Read the model definition and answer for the solid it produces. Units are mm, in the model's axes. A direction names the side the tool comes from. Give positions to 0.01 mm unless a question says otherwise; leave off trailing zeros. Loops run counter-clockwise (first coordinate to the right, second up) from the corner with the lowest first, then second, coordinate; pieces in that order, holes last. Notation, with made-up numbers: (9, 13.25) -> (30, 13.25) arc R30 cw to (30, 49.25) -> close; hole circle Ø1 at (-16.75, 30). An arc over 180 degrees is marked (long way). Return JSON: item names as keys, results as strings. Group by question number.
from build123d import *

# Parameters (mm, degrees)
SKETCH1_R           = 400
BOSS_EXTRUDE1_DEPTH = 200
BOSS_EXTRUDE2_START = -10
SKETCH2_R           = 82.5
SKETCH2_R_2         = 75.5
BOSS_EXTRUDE2_DEPTH = 33
CUT_EXTRUDE1_START  = -432
SKETCH2_2_R         = 75.5
CUT_EXTRUDE1_DEPTH  = 432
SKETCH3_R           = 275.958825931
CUT_EXTRUDE3_DEPTH  = 175
FILLET2_R           = 10


with BuildPart() as part:
    # Sketch1 → Boss-Extrude1 (new body)
    with BuildSketch(Plane(origin=(0, 0, 0), x_dir=(1, 0, 0), z_dir=(0, 1, 0))):
        with Locations(Location((0, 0, 0), (0, 0, 270))):
            Circle(SKETCH1_R)
    extrude(amount=BOSS_EXTRUDE1_DEPTH)

    # Sketch2 → Boss-Extrude2 (add)
    with BuildSketch(Plane.XY.offset(400).offset(BOSS_EXTRUDE2_START)):
        with Locations(Location((0, 104.933431854, 0), (0, 0, 180))):
            Circle(SKETCH2_R)
        with Locations(Location((0, 104.933431854, 0), (0, 0, 180))):
            Circle(SKETCH2_R_2, mode=Mode.SUBTRACT)
    extrude(amount=BOSS_EXTRUDE2_DEPTH)

    # Sketch2_2 → Cut-Extrude1 (cut)
    with BuildSketch(Plane.XY.offset(400).offset(CUT_EXTRUDE1_START)):
        with Locations((0, 104.933431854)):
            Circle(SKETCH2_2_R)
    extrude(amount=CUT_EXTRUDE1_DEPTH, mode=Mode.SUBTRACT)

    # Sketch3 → Cut-Extrude3 (cut)
    with BuildSketch(Plane(origin=(0, 200, 0), x_dir=(1, 0, 0), z_dir=(0, 1, 0))):
        with Locations(Location((0, 0, 0), (0, 0, 270))):
            Circle(SKETCH3_R)
    extrude(amount=-CUT_EXTRUDE3_DEPTH, mode=Mode.SUBTRACT)

    # Fillet2
    fillet2_edges = [part.edges().sort_by_distance(p)[0] for p in [
        (82.5, 104.933431854, 391.399731732),
    ]]
    fillet(fillet2_edges, radius=FILLET2_R)


solid = part.part
1. Flat-ended cylindrical pins translate along their axes: pin 1 Ø1.5 at (y, z) = (149.5, -123) entering from +X; pin 2 Ø3 at (x, y) = (-198, 95.5) entering from -Z; pin 3 Ø6 at (y, z) = (159.5, 250) entering from +X. Find the tip coordinate at first contact, or state that the pin passes through.
2. Section B-B on x = 132 is taken. Determine the outline of the cut face in (y, z).
3. Which of the six approach directions +Z, -Z, +X, -X, +Y, -Y give full straight-line access (tool end or side, diameter ignored) to faces 5 (the flat face through (6, 0, -6)), 6 (the cylindrical face through (4.98, 180.27, 343.11))?
4. Section C-C on x = -321.5 is taken. Determine the outline of the cut face in (y, z).
5. Straight lines are drawn through the part: line 1 (X direction, y = 118, z = 0); line 2 (Z direction, x = -170.5, y = 40); line 3 (Y direction, x = 0, z = 344.5). For each, find the intervals that lie inside material, in ascending order. Write a range as from..to.
6. Section A-A on z = 0 is taken. Determine the outline of the cut face in (x, y).
7. Determine the mould class of faces 1 (the cylindrical face through (82.891, 113.725, 263.216)), 2 (the flat face through (94, 200, 261)), 3 (the flat face through (4, 25, -4)), 4 (the flat face through (-36, 172, 423)) for opening direction Z: pulls with the +Z half, pulls with the -Z half, needs draft (parallel to the pull), parting line crosses it, or undercut.
Completed:
{
 "1": {"pin 1": "stops at x = 380.86", "pin 2": "stops at z = -348.41", "pin 3": "stops at x = 314.63"},
 "2": {"outline": "(0, -377.59) -> (200, -377.59) -> (200, -242.34) -> (25, -242.34) -> (25, 242.34) -> (200, 242.34) -> (200, 377.59) -> (0, 377.59) -> close"},
 "3": {"face 5": "+Z, -Z, +X, -X, -Y", "face 6": "+Z"},
 "4": {"outline": "(0, -237.99) -> (200, -237.99) -> (200, 237.99) -> (0, 237.99) -> close"},
 "5": {"line 1": "x = -400..-275.96, 275.96..400", "line 2": "z = -361.84..-216.99, 216.99..361.84", "line 3": "y = 0..29.43, 180.43..200"},
 "6": {"outline": "(-400, 0) -> (400, 0) -> (400, 200) -> (275.96, 200) -> (275.96, 25) -> (-275.96, 25) -> (-275.96, 200) -> (-400, 200) -> close"},
 "7": {"face 1": "undercut", "face 2": "needs draft", "face 3": "undercut", "face 4": "pulls with the +Z half"}
}
